Source: CAD feature listing. Evaluate the final solid. Frame: model axes, mm. A direction names the side the tool comes from. Round coordinates to 2 decimals unless told otherwise and drop trailing zeros. Loops run counter-clockwise (first coordinate to the right, second up) from the corner with the lowest first, then second, coordinate; pieces in that order, holes last.
Item 1: Pull-direction query (Y, two-part tool) for faces 3 (the cylindrical face through (-12.7, -5.13, 2.46)), 4 (the flat face through (-11, -4, 5)), 5 (the cylindrical face through (-22.2, 5.3, 0.1)); classes: released by +Y, released by -Y, zero draft, split by the parting line, or undercut.
Item 2: Section query C-C on x = 0.75. Return loops of the section in (y, z).
Item 3: Section query B-B on z = 4. Return loops of the section in (x, y).
Item 4: Ray query, L1, parallel to Y at x = -12.5, z = 0.75; L2, parallel to X at y = -7.25, z = 3.25; L3, parallel to X at y = -17.5, z = 2. Return the intervals inside material, ascending.
Item 5: First-contact query: P1, Ø4, axis at x = -10.85, y = -6.82, coming from the +Z side. Flat tip, straight axial feed; report the tip coordinate or a pass-through.
Item 6: Section query A-A on x = -11. Return loops of the section in (y, z), then the cut area to 3 significant figures.
Item 7: Access query for faces 1 (the flat face through (-11, -7, 0)), 2 (the cylindrical face through (1.345, 5.268, 0.07)). Directions: +Z, -Z, +X, -X, +Y, -Y. A direction counts if a zero-diameter tool reaches every point of the face in a straight line with its end or side. Return the directions, or none.
```python
from build123d import *

# Parameters (mm, degrees)
F0_R     = 2.5
F1_DEPTH = 4.9999998882
F2_DEPTH = 5


with BuildPart() as f1:
    # F0 (on Top) → F1 (new body)
    with BuildSketch(Plane.XY):
        with BuildLine():
            Line((-0.4416928518, 6.0201503709), (-20.4416928518, 6.0201503709))
            ThreePointArc((-20.4416928518, 6.0201503709), (-22.2094598048, 5.2879173239), (-22.9416928518, 3.5201503709))
            Line((-22.9416928518, 3.5201503709), (-22.9416928518, -16.4798496291))
            ThreePointArc((-22.9416928518, -16.4798496291), (-22.2094598048, -18.2476165821), (-20.4416928518, -18.9798496291))
            Line((-20.4416928518, -18.9798496291), (-0.4416928518, -18.9798496291))
            ThreePointArc((-0.4416928518, -18.9798496291), (1.3260741011, -18.2476165821), (2.0583071482, -16.4798496291))
            Line((2.0583071482, -16.4798496291), (2.0583071482, 3.5201503709))
            ThreePointArc((2.0583071482, 3.5201503709), (1.3260741011, 5.2879173239), (-0.4416928518, 6.0201503709))
        make_face()
        with Locations((-10.8535308391, -6.8182437681)):
            Circle(F0_R, mode=Mode.SUBTRACT)
    extrude(amount=F1_DEPTH)

    # F0 (on Top) → F2 (join)
    with BuildSketch(Plane.XY):
        with BuildLine():
            Line((-0.4416928518, 6.0201503709), (-20.4416928518, 6.0201503709))
            ThreePointArc((-20.4416928518, 6.0201503709), (-22.2094598048, 5.2879173239), (-22.9416928518, 3.5201503709))
            Line((-22.9416928518, 3.5201503709), (-22.9416928518, -16.4798496291))
            ThreePointArc((-22.9416928518, -16.4798496291), (-22.2094598048, -18.2476165821), (-20.4416928518, -18.9798496291))
            Line((-20.4416928518, -18.9798496291), (-0.4416928518, -18.9798496291))
            ThreePointArc((-0.4416928518, -18.9798496291), (1.3260741011, -18.2476165821), (2.0583071482, -16.4798496291))
            Line((2.0583071482, -16.4798496291), (2.0583071482, 3.5201503709))
            ThreePointArc((2.0583071482, 3.5201503709), (1.3260741011, 5.2879173239), (-0.4416928518, 6.0201503709))
        make_face()
        with Locations((-10.8535308391, -6.8182437681)):
            Circle(F0_R, mode=Mode.SUBTRACT)
        with Locations((-10.8535308391, -6.8182437681)):
            Circle(F0_R)
    extrude(amount=-F2_DEPTH)


solid = f1.part
```
Data:
1. face 3: undercut
1. face 4: zero draft
1. face 5: released by +Y
2. outline: (-18.68, -5) - (5.72, -5) - (5.72, 5) - (-18.68, 5) - close
3. outline: (-22.94, -16.48) arc R2.5 ccw to (-20.44, -18.98) - (-0.44, -18.98) arc R2.5 ccw to (2.06, -16.48) - (2.06, 3.52) arc R2.5 ccw to (-0.44, 6.02) - (-20.44, 6.02) arc R2.5 ccw to (-22.94, 3.52) - close; hole circle Ø5 at (-10.85, -6.82)
4. L1: y = -18.98 to -8.7, -4.94 to 6.02
4. L2: x = -22.94 to -13.32, -8.39 to 2.06
4. L3: x = -22.72 to 1.84
5. P1: stops at z = 0
6. outline: (-18.98, -5) - (6.02, -5) - (6.02, 5) - (-4.32, 5) - (-4.32, 0) - (-9.31, 0) - (-9.31, 5) - (-18.98, 5) - close
6. area: 225 mm2
7. face 1: +Z
7. face 2: +Z, -Z, +X, +Y
